Answer from the drawing. Dimensions are ordinates in mm from the lowest x, y and z of the part. Give positions to 0.01 mm unless a question says otherwise; leave off trailing zeros. Order: outer loops, then holes, each group sorted by start corner. A loop starts at its lowest first (then second) coordinate and runs counter-clockwise, first axis right, second up. Notation, with made-up numbers: (27, -32.5) - (56, -32.5) arc R22 cw to (56, 5.5) - close; hole circle Ø10 at (61.25, 71). An arc over 180 degrees is marked (long way). Answer in a Markdown table with one row per item.
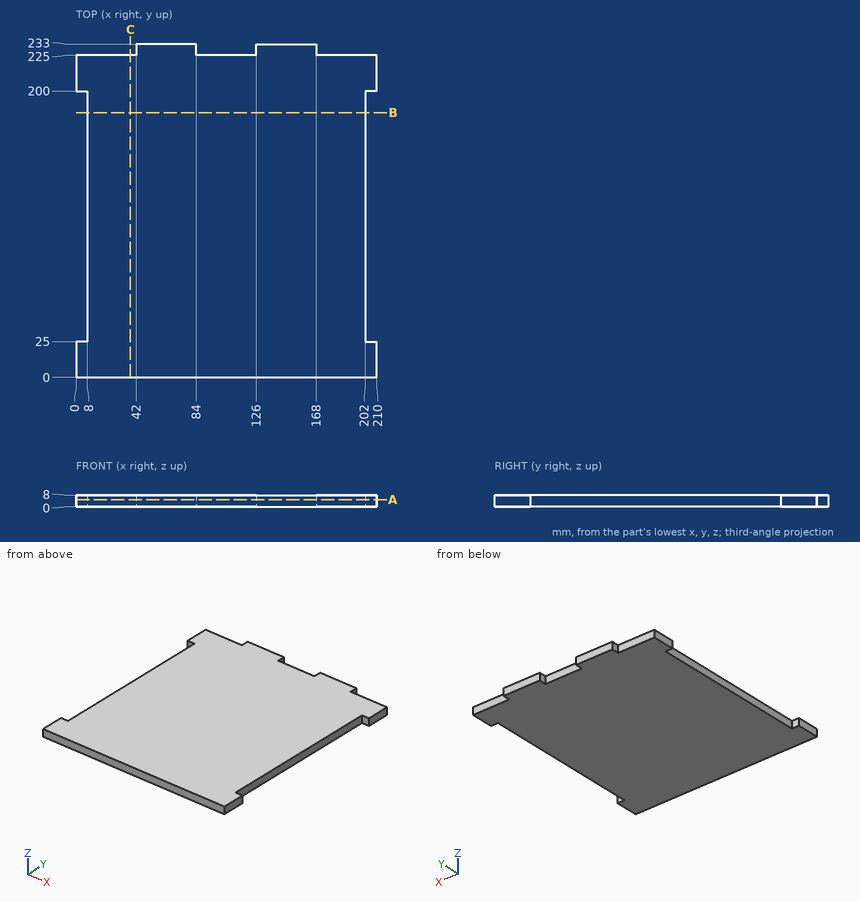
Item 1: Find section C-C on x = 38. Write down the section's boundary in (y, z), then the cut area to 3 significant figures.
Answer block:
| item | result |
|---|---|
| outline | (0, 0) - (225, 0) - (225, 8) - (0, 8) - close |
| area | 1,800 mm² |
Item 2: Find section A-A on z = 5. Write down the section's boundary in (x, y), then the cut area to 3 significant figures.
Answer block:
| item | result |
|---|---|
| outline | (0, 0) - (210, 0) - (210, 25) - (202, 25) - (202, 200) - (210, 200) - (210, 225) - (168, 225) - (168, 233) - (126, 233) - (126, 225) - (84, 225) - (84, 233) - (42, 233) - (42, 225) - (0, 225) - (0, 200) - (8, 200) - (8, 25) - (0, 25) - close |
| area | 45,100 mm² |
Item 3: Consider line 1 (X direction, y = 28.5, z = 3); line 2 (Y direction, x = 124.5, z = 4.5). Determine where each line is inside the solid, lowest interval first.
Answer block:
| item | result |
|---|---|
| line 1 | 8 to 202 |
| line 2 | 0 to 225 |
Item 4: Each of these flat-tipped pins is pushed along its axis until it touches: P1, Ø1.5, axis at x = 63.5, z = 4, coming from the -Y side; P2, Ø4, axis at y = 142, z = 5.5, coming from the -X side; P3, Ø2, axis at x = 101, z = 3, coming from the +Y side; P4, Ø2.5, axis at y = 104, z = 3, coming from the +X side. Where does it stop, or does it pass through?
Answer block:
| item | result |
|---|---|
| P1 | y = 0 |
| P2 | x = 8 |
| P3 | y = 225 |
| P4 | x = 202 |
Item 5: Find section B-B on y = 185. Write down the section's boundary in (x, z), then the cut area to 3 significant figures.
Answer block:
| item | result |
|---|---|
| outline | (8, 0) - (202, 0) - (202, 8) - (8, 8) - close |
| area | 1,550 mm² |
